Can you work these out from the model? Positions are in its coordinate system, mm. Coordinates: 2 decimals unless noted, no trailing zeros. Write each loop counter-clockwise with the first axis right and the second up, starting at its lowest first coordinate (ties: lowest second). Pieces come first, ordered by that corner, then holes. Notation, with made-up numbers: (-24.75, -2.5) - (31.25, -2.5) arc R34 cw to (31.25, 33.5) - close; hole circle Ø3 at (9, 2). An arc over 180 degrees is marked (long way). Use one line per item in the form item = value. Start each with the question number.
(1) If I drill on probe 1 along Z at (x, y) = (-98, 4.35); probe 2 along X at (y, z) = (0.9, -5); probe 3 along Z at (x, y) = (-15, 2.9), over which ranges is the centre line in solid material (lowest first)? Write a range as from..to.
(2) If we section it at C-C on x = -50: Please give me the cut outline in (y, z).
(3) If we section it at B-B on z = 19.5: Please give me the cut outline in (x, y), then the cut area to 3 significant figures.
(4) If we section it at A-A on y = 1.1: Please give me the cut outline in (x, z) (3 decimals).
(5) If we section it at D-D on z = -2: Give the number of separate pieces and of enclosed holes in the cut face, then the cut area to 3 significant figures.
(6) Thinking about a two-plate mould opening in Z: for faces 1 (the face through (-48, 0, 53)), 2 (the face through (9.22, 2.5, -8.73)), which applies, pulls with the +Z half, pulls with the -Z half, needs draft (parallel to the pull), parting line crosses it, or undercut?
(7) For pin 1 Ø2 at (x, y) = (-63, 2) entering from +Z; pin 2 Ø1.5 at (x, y) = (-4.5, 1) entering from +Z; pin 3 Ø4 at (x, z) = (3.8, 58.21) entering from +Y; pin 4 Ø7.5 at (x, z) = (-97.5, -2.25) entering from +Y, each with a flat end and sliding along its axis, tell me the tip position at first contact or that it passes through.
```python
from build123d import *

# Parameters (mm, degrees)
SKETCH1_R           = 3.175
BOSS_EXTRUDE1_DEPTH = 5.08
SKETCH2_W           = 7.62
SKETCH2_H           = 5.08
REVOLVE1_ANGLE      = 180
SKETCH3_W           = 7.62
SKETCH3_H           = 5.08
REVOLVE2_ANGLE      = 180
SKETCH4_R           = 2.54
CUT_EXTRUDE1_DEPTH  = 161.661116131
SKETCH5_R           = 2.54
CUT_EXTRUDE2_DEPTH  = 161.661116131
FILLET1_R           = 3.175


with BuildPart() as part:
    # Sketch1 → Boss-Extrude1 (new body)
    with BuildSketch(Plane(origin=(0, 0, 0), x_dir=(1, 0, 0), z_dir=(0, 1, 0))):
        with BuildLine():
            Line((-7.011572103, 0), (-88.238427897, 0))
            ThreePointArc((-88.238427897, 0), (-104.230256121, 8.980256121), (-95.25, -7.011572103))
            Line((-95.25, -7.011572103), (-95.25, -100.938427897))
            ThreePointArc((-95.25, -100.938427897), (-104.230256121, -116.930256121), (-88.238427897, -107.95))
            Line((-88.238427897, -107.95), (-7.011572103, -107.95))
            ThreePointArc((-7.011572103, -107.95), (8.980256121, -116.930256121), (0, -100.938427897))
            Line((0, -100.938427897), (0, -7.011572103))
            ThreePointArc((0, -7.011572103), (8.980256121, 8.980256121), (-7.011572103, 0))
        make_face()
        with Locations(Location((-97.49506403, 2.24506403, 0), (0, 0, 270))):
            Circle(SKETCH1_R, mode=Mode.SUBTRACT)
        with Locations(Location((2.24506403, 2.24506403, 0), (0, 0, 270))):
            Circle(SKETCH1_R, mode=Mode.SUBTRACT)
        with Locations(Location((2.24506403, -110.19506403, 0), (0, 0, 270))):
            Circle(SKETCH1_R, mode=Mode.SUBTRACT)
        with Locations(Location((-97.49506403, -110.19506403, 0), (0, 0, 270))):
            Circle(SKETCH1_R, mode=Mode.SUBTRACT)
    extrude(amount=BOSS_EXTRUDE1_DEPTH)

    # Sketch2 → Revolve1 (revolve)
    with BuildSketch(Plane.ZY.offset(95.25)):
        with Locations((53.34, 2.54)):
            Rectangle(SKETCH2_W, SKETCH2_H)
    revolve(axis=Axis((-95.25, 5.08, 49.53), (0, -1, 0)), revolution_arc=REVOLVE1_ANGLE)

    # Sketch3 → Revolve2 (revolve)
    with BuildSketch(Plane(origin=(0, 0, 0), x_dir=(0, 0, -1), z_dir=(1, 0, 0))):
        with Locations((-62.23, 2.54)):
            Rectangle(SKETCH3_W, SKETCH3_H)
    revolve(axis=Axis((0, 5.08, 58.42), (0, 1, 0)), revolution_arc=REVOLVE2_ANGLE)

    # Sketch4 → Cut-Extrude1 (cut, through all)
    with BuildSketch(Plane(origin=(0, 5.08, 0), x_dir=(1, 0, 0), z_dir=(0, 1, 0))):
        with Locations(Location((-99.053632383, -49.309816677, 0), (0, 0, 270))):
            Circle(SKETCH4_R)
    extrude(amount=-CUT_EXTRUDE1_DEPTH, mode=Mode.SUBTRACT)

    # Sketch5 → Cut-Extrude2 (cut, through all)
    with BuildSketch(Plane(origin=(0, 5.08, 0), x_dir=(1, 0, 0), z_dir=(0, 1, 0))):
        with Locations(Location((3.804450658, -58.214439329, 0), (0, 0, 270))):
            Circle(SKETCH5_R)
    extrude(amount=-CUT_EXTRUDE2_DEPTH, mode=Mode.SUBTRACT)

    # Fillet1
    fillet1_edges = [part.edges().sort_by_distance(p)[0] for p in [
        (-97.49506403, 5.08, -5.42006403),
        (2.24506403, 5.08, -5.42006403),
        (2.24506403, 5.08, 107.02006403),
        (-97.49506403, 5.08, 107.02006403),
    ]]
    fillet(fillet1_edges, radius=FILLET1_R)


solid = part.part
```
Reported:
q1.probe_1 = -11.76..-6.54, 2.05..7.27, 42.42..47, 51.62..56.64, 100.68..105.9, 114.49..119.71
q1.probe_2 = -106.61..-99.07, -95.92..-88.38, -6.87..0.67, 3.82..11.36
q1.probe_3 = 0..107.95
q2.outline = (0, 0) - (5.08, 0) - (5.08, 107.95) - (0, 107.95) - close
q3.outline = (-95.25, 0) - (0, 0) - (0, 5.08) - (-95.25, 5.08) - close
q3.area = 484 mm2
q4.outline = (-95.25, 7.012) arc R9.525 ccw (long way) to (-88.238, 0) - (-7.012, 0) arc R9.525 ccw (long way) to (0, 7.012) - (0, 50.8) arc R7.62 ccw to (0, 66.04) - (0, 100.938) arc R9.525 ccw (long way) to (-7.012, 107.95) - (-88.238, 107.95) arc R9.525 ccw (long way) to (-95.25, 100.938) - (-95.25, 57.15) arc R7.62 ccw to (-95.25, 41.91) - close; hole circle Ø5.08 at (-99.054, 49.31); hole circle Ø6.35 at (-97.495, -2.245); hole circle Ø6.35 at (-97.495, 110.195); hole circle Ø6.35 at (2.245, -2.245); hole circle Ø6.35 at (2.245, 110.195); hole circle Ø5.08 at (3.804, 58.214)
q5.separate_pieces = 4
q5.enclosed_holes = 0
q5.area = 120 mm2
q6.face_1 = needs draft
q6.face_2 = undercut
q7.pin_1 = 107.95
q7.pin_2 = 117.6
q7.pin_3 = through
q7.pin_4 = 3.74
